For this review, take the finished solid that the model builds, in its own axes (mm). Face numbers are marked on the shaded views. A direction names the side the tool comes from. Round coordinates to 2 decimals unless told otherwise and drop trailing zeros. Loops run counter-clockwise (first coordinate to the right, second up) from the corner with the lowest first, then second, coordinate; pieces in that order, holes last. Notation, with made-up numbers: (44, 23.25) -> (48, 23.25) arc R23 cw to (48, 38.25) -> close; hole circle Ø2 at (55, 82). An arc over 180 degrees is marked (long way). Use one line per item in the form item = value. Start each with the question number.
from build123d import *

# Parameters (mm, degrees)
CROQUIS1_R              = 17.5
SALIENTE_EXTRUIR1_DEPTH = 12.5
CROQUIS2_R              = 6
SALIENTE_EXTRUIR2_DEPTH = 72.5


with BuildPart() as part:
    # Croquis1 → Saliente-Extruir1 (new body, symmetric)
    with BuildSketch(Plane(origin=(0, 0, 0), x_dir=(0, 0, -1), z_dir=(1, 0, 0))):
        Circle(CROQUIS1_R)
    extrude(amount=SALIENTE_EXTRUIR1_DEPTH, both=True)

    # Croquis2 → Saliente-Extruir2 (add)
    with BuildSketch(Plane(origin=(12.5, 0, 0), x_dir=(0, 0, -1), z_dir=(1, 0, 0))):
        Circle(CROQUIS2_R)
    saliente_extruir2 = extrude(amount=SALIENTE_EXTRUIR2_DEPTH)

    # Simetría1: Saliente-Extruir2 across plane
    add(saliente_extruir2.mirror(Plane(origin=(0, 0, 0), x_dir=(0, 0, 1), z_dir=(1, 0, 0))))


solid = part.part
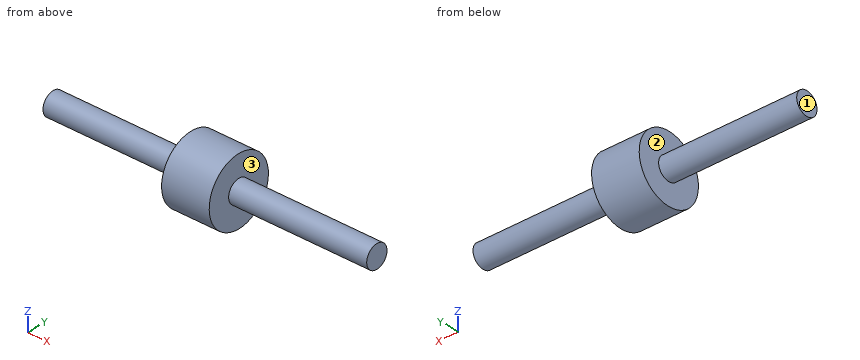
Item 1: Take a section at C-C on x = -20. Give the boundary of the cut face in (y, z), plus the area to 3 significant figures.
Item 2: Wall thickness on line 1 (X direction, y = -10, z = 2); line 2 (Z direction, x = 71, y = -0.5); line 3 (Y direction, x = 0, z = 9.5): over which ranges is each line inside the solid? List them lowest first.
Item 3: Machinability: for the marked faces 1, 2 and 3, which of the approach directions +Z, -Z, +X, -X, +Y, -Y give a long, thin tool a straight path to every point of the face, cutting with its end or side? Answer none if there is none.
Item 4: Take a section at A-A on y = 0. Give the boundary of the cut face in (x, z), plus the area to 4 significant figures.
Item 5: For P1, Ø10, axis at x = 40, y = -7, coming from the +Z side; P2, Ø5, axis at y = 1, z = -13.5, coming from the -X side; P3, Ø12, axis at x = -5, y = 10, coming from the -Z side, all flat-tipped, find the tip position at first contact; note any pin that passes through.
Item 6: Take a section at D-D on x = 10. Give the boundary of the cut face in (y, z).
Results:
q1.outline = circle Ø12 at (0, 0)
q1.area = 113 mm2
q2.line_1 = -12.5 to 12.5
q2.line_2 = -5.98 to 5.98
q2.line_3 = -14.7 to 14.7
q3.face_1 = +Z, -Z, -X, +Y, -Y
q3.face_2 = -X
q3.face_3 = +X
q4.outline = (-85, -6) -> (-12.5, -6) -> (-12.5, -17.5) -> (12.5, -17.5) -> (12.5, -6) -> (85, -6) -> (85, 6) -> (12.5, 6) -> (12.5, 17.5) -> (-12.5, 17.5) -> (-12.5, 6) -> (-85, 6) -> close
q4.area = 2,615 mm2
q5.P1 = 5.66
q5.P2 = -12.5
q5.P3 = -17.04
q6.outline = circle Ø35 at (0, 0)
